Model file for the job. Use its own axes, mm. Give positions to 0.01 mm unless a question says otherwise; leave off trailing zeros. Write each loop counter-clockwise with the first axis right and the second up, starting at its lowest first coordinate (ties: lowest second). Pieces come first, ordered by that corner, then holes. Notation, with made-up numbers: M -21.75,13 L 15.25,13 A10 cw 15.25,22 Z; hole C -16.5,37.5 d1. An arc over 180 degrees is marked long. Answer as a JSON object with one key per item and string values. Group by question number.
```python
from build123d import *

# Parameters (mm, degrees)
F2_R     = 6.115272
F4_DEPTH = 15.7


with BuildPart() as f1:
    # F0 (on Top) → F1 (revolve)
    with BuildSketch(Plane.XY):
        Polygon((0, -25.548944), (0, 18.719036), (-31.367026, 18.719036), align=None)
    revolve(axis=Axis((0, -3.414954, 0), (0, 1, 0)))

    # F2
    f2_edges = [f1.edges().sort_by_distance(p)[0] for p in [
        (31.367026, 18.719036, 0),
    ]]
    fillet(f2_edges, radius=F2_R)

    # F3 (on face) → F4 (cut)
    with BuildSketch(Plane(origin=(0, 18.719036, 0), x_dir=(-1, 0, 0), z_dir=(0, 1, 0))):
        Polygon((-0.096357, 5.727981), (-5.008755, 2.780543), (-4.912399, -2.947438), (0.096357, -5.727981), (5.008755, -2.780543), (4.912399, 2.947438), align=None)
    extrude(amount=-F4_DEPTH, mode=Mode.SUBTRACT)


solid = f1.part
```
Q1. Two-plate mould, pull along Z, no slides. Class faces 1 (the flat face through (-2.518, 10.979, -4.275)), 2 (the flat face through (4, 18.719, -4)), 3 (the conical face through (2.031, -12.329, -9.145)): +Z half, -Z half, draft (parallel to the pull), parting line (faces both ways), or undercut.
Q2. Slice it at A-A, the plane y = -5.5. Write the cut outline in (x, z).
Q3. Wall check: L1, parallel to X at y = 16, z = 15; L2, parallel to X at y = 4, z = 4.5; L3, parallel to X at y = 7.5, z = -2.5. Give the ranges that are in metal, low to high.
Q4. Drop flat-ended pins along their axis: P1, Ø2, axis at y = -1.5, z = -10, coming from the +X side; P2, Ø1.5, axis at x = -10, y = -0.5, coming from the -Z side; P3, Ø10, axis at x = 3, y = -18, coming from the -Z side. Give the stop position or say it passes through.
Q5. Slice it at B-B, the plane y = -21.5. Write the cut outline in (x, z).
Solved:
{
 "1": {"face 1": "undercut", "face 2": "draft", "face 3": "parting line"},
 "2": {"outline": "C 0,0 d28.41"},
 "3": {"L1": "x = -19.53 to 19.53", "L2": "x = -20.45 to -2.12, 2.14 to 20.45", "L3": "x = -23.28 to -5, 4.92 to 23.28"},
 "4": {"P1": "stops at x = 14.89", "P2": "stops at z = -15.46", "P3": "stops at z = -8.6"},
 "5": {"outline": "C 0,0 d5.74"}
}
